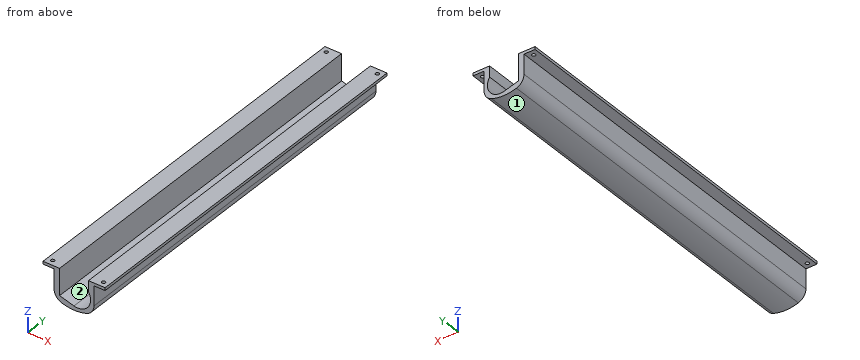
```python
from build123d import *

# Parameters (mm, degrees)
BOSS_EXTRUDE1_DEPTH = 431.8
FILLET2_R           = 12.7
SKETCH2_R           = 2.032
CUT_EXTRUDE1_DEPTH  = 436.166892099


with BuildPart() as part:
    # Sketch1 → Boss-Extrude1 (new body)
    with BuildSketch(Plane(origin=(0, 0, 0), x_dir=(1, 0, 0), z_dir=(0, 1, 0))):
        with BuildLine():
            Line((12.446, -95.666893232), (12.446, -83.267976842))
            ThreePointArc((12.446, -83.267976842), (12.103082443, -66.082532596), (-4.162019583, -60.523437125))
            Line((-4.162019583, -60.523437125), (-20.574, -65.268050741))
            Line((-20.574, -65.268050741), (-20.574, -84.572180345))
            Line((-20.574, -84.572180345), (-20.574, -95.666893232))
            Line((-20.574, -95.666893232), (-39.624, -95.666893232))
            Line((-39.624, -95.666893232), (-39.624, -92.491893232))
            Line((-39.624, -92.491893232), (-26.924, -92.491893232))
            Line((-26.924, -92.491893232), (-26.924, -62.093050741))
            ThreePointArc((-26.924, -62.093050741), (-4.064, -55.764211531), (18.796, -62.093050741))
            Line((18.796, -62.093050741), (18.796, -92.491893232))
            Line((18.796, -92.491893232), (31.496, -92.491893232))
            Line((31.496, -92.491893232), (31.496, -95.666893232))
            Line((31.496, -95.666893232), (12.446, -95.666893232))
        make_face()
    extrude(amount=BOSS_EXTRUDE1_DEPTH)

    # Fillet2
    fillet2_edges = [part.edges().sort_by_distance(p)[0] for p in [
        (-26.924, 215.9, 62.093050741),
        (18.796, 215.9, 62.093050741),
    ]]
    fillet(fillet2_edges, radius=FILLET2_R)

    # Sketch2 → Cut-Extrude1 (cut, through all)
    with BuildSketch(Plane(origin=(0, 0, 92.491893232), x_dir=(-1, 0, 0), z_dir=(0, 0, -1))):
        with Locations((-25.146, 425.45)):
            Circle(SKETCH2_R)
        with Locations((-25.146, 6.35)):
            Circle(SKETCH2_R)
        with Locations((33.274, 425.45)):
            Circle(SKETCH2_R)
        with Locations((33.274, 6.35)):
            Circle(SKETCH2_R)
    extrude(amount=-CUT_EXTRUDE1_DEPTH, mode=Mode.SUBTRACT)


solid = part.part
```
Work out the finished part from the listing and answer in its coordinate system (mm). Face numbers are marked on the shaded views. Coordinates: 2 decimals unless noted, no trailing zeros. Write each loop counter-clockwise with the first axis right and the second up, starting at its lowest first coordinate (ties: lowest second). Pieces come first, ordered by that corner, then holes.
Q1. A cutting plane is placed at B-B, the plane y = 71.5. Give the vertices of the cut face in (x, z), then the cut area to 3 significant figures.
Q2. Determine the mould class of the marked faces 1 and 2 for opening direction X: released by +X, released by -X, zero draft, split by the parting line, or undercut.
Q3. Find the intervals of material crossed by line 1 (X direction, y = 266, z = 76.5); line 2 (X direction, y = 94, z = 89); line 3 (Z direction, x = 28, y = 67.5), in increasing order.
Q4. Each of these flat-tipped pins is pushed along its axis until it touches: pin 1 Ø6 at (y, z) = (166, 91.5) entering from -X; pin 2 Ø5 at (y, z) = (118.5, 79.5) entering from -X; pin 3 Ø3.5 at (x, y) = (25.146, 6.35) entering from +Z; pin 4 Ø6 at (y, z) = (322.5, 85.5) entering from +X. Where does it stop, or does it pass through?
Q5. A cutting plane is placed at C-C, the plane x = 6. Give the vertices of the cut face in (y, z), then the cut area to 3 significant figures.
Q6. A cutting plane is placed at A-A, the plane z = 74. Give the vertices of the cut face in (x, y).
Findings below:
1. outline: (-39.62, 92.49) - (-26.92, 92.49) - (-26.92, 70.13) arc R12.7 ccw to (-18.29, 58.1) arc R44.45 ccw to (10.16, 58.1) arc R12.7 ccw to (18.8, 70.13) - (18.8, 92.49) - (31.5, 92.49) - (31.5, 95.67) - (12.45, 95.67) - (12.45, 83.27) arc R14.99 cw to (-4.16, 60.52) - (-20.57, 65.27) - (-20.57, 95.67) - (-39.62, 95.67) - close
1. area: 652 mm2
2. face 1: split by the parting line
2. face 2: undercut
3. line 1: x = -26.92 to -20.57, 14.9 to 18.8
3. line 2: x = -26.92 to -20.57, 12.45 to 18.8
3. line 3: z = 92.49 to 95.67
4. pin 1: stops at x = -39.62
4. pin 2: stops at x = -26.92
4. pin 3: passes through
4. pin 4: stops at x = 18.8
5. outline: (0, 56.92) - (431.8, 56.92) - (431.8, 61.19) - (0, 61.19) - close
5. area: 1,840 mm2
6. outline: (-26.92, 0) - (-20.57, 0) - (-20.57, 431.8) - (-26.92, 431.8) - close; (14.96, 0) - (18.8, 0) - (18.8, 431.8) - (14.96, 431.8) - close
